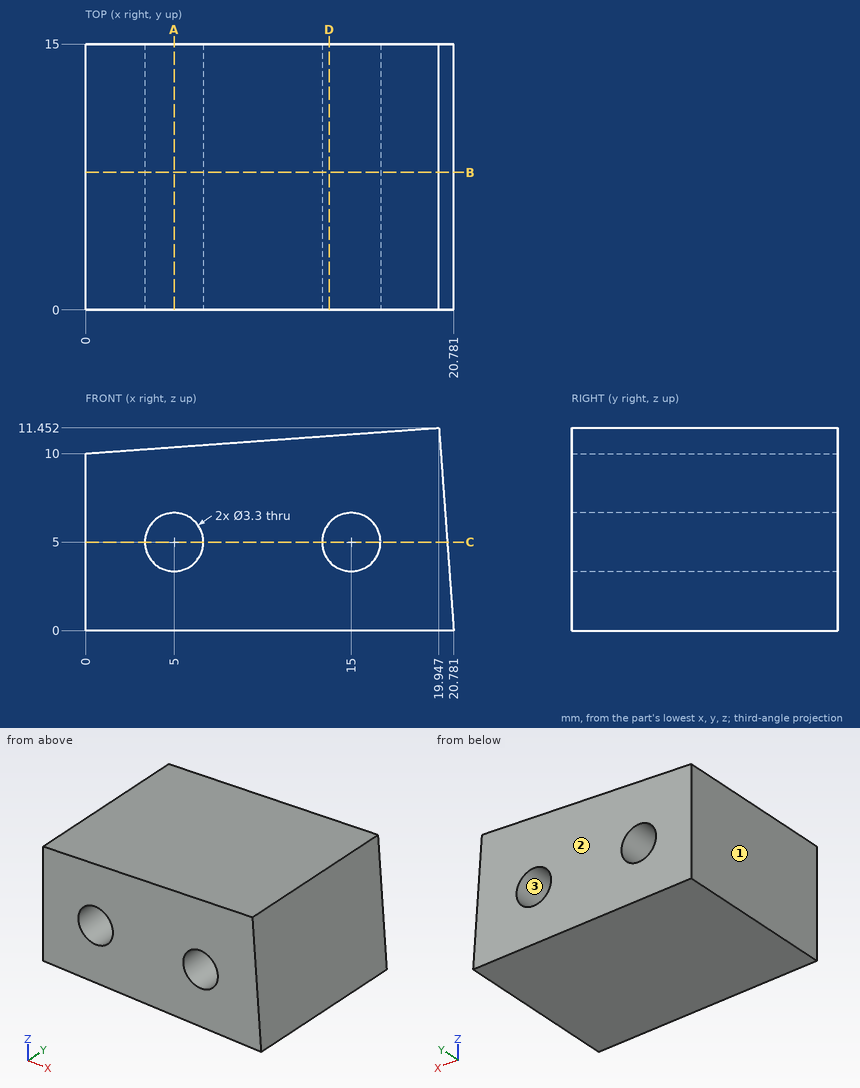
Design review of the part shown in the three views and the two pictorial views. Dimensions are in mm from the part's minimum x, y and z. Round coordinates to 2 decimals unless told otherwise and drop trailing zeros. Write each loop counter-clockwise with the first axis right and the second up, starting at its lowest first coordinate (ties: lowest second). Pieces come first, ordered by that corner, then holes. Notation, with made-up numbers: M 75,47.25 L 95,47.25 A16 cw 95,53.25 Z; hole C -22.75,62.25 d3. An arc over 180 degrees is marked long. One line per item, written item: value. Start each with the question number.
1. Take a section at A-A on x = 5. State the section outline as (y, z) points, then the cut area to 3 significant figures.
2. Take a section at C-C on z = 5. State the section outline as (x, y) points, then the cut area to 3 significant figures.
3. Draft analysis for pull direction X (two halves, no side actions). For the marked faces 1, 2 and 3, state which applies: pulls with the +X half, pulls with the -X half, needs draft (parallel to the pull), parting line crosses it, or undercut.
4. To check wall thickness, follow probe 1 along X at (y, z) = (4, 5); probe 2 along X at (y, z) = (11.25, 6.5) (1 decimal); probe 3 along Z at (x, y) = (4, 0.75). State the ranges of each line that lie inside material, in increasing order. Write a range as from..to.
5. Clearance check with flat-ended pins moving along their axes: P1, Ø1, axis at x = 5, y = 1.5, coming from the +Z side; P2, Ø4, axis at x = 10, y = 12, coming from the +Z side; P3, Ø5, axis at x = 9, y = 7, coming from the +Z side; P4, Ø2.5, axis at x = 15, z = 5, coming from the +Y side. State where each tip first meets the part, or that it passes through.
6. Take a section at D-D on x = 13.75. State the section outline as (y, z) points.
7. Take a section at B-B on y = 7.75. State the section outline as (x, z) points, then the cut area to 3 significant figures.
Computed:
1. outline: M 0,0 L 15,0 L 15,3.35 L 0,3.35 Z; M 0,6.65 L 15,6.65 L 15,10.36 L 0,10.36 Z
1. area: 106 mm²
2. outline: M 0,0 L 3.35,0 L 3.35,15 L 0,15 Z; M 6.65,0 L 13.35,0 L 13.35,15 L 6.65,15 Z; M 16.65,0 L 20.42,0 L 20.42,15 L 16.65,15 Z
2. area: 207 mm²
3. face 1: pulls with the -X half
3. face 2: needs draft
3. face 3: undercut
4. probe 1: x = 0..3.35, 6.65..13.35, 16.65..20.42
4. probe 2: x = 0..4.3, 5.7..14.3, 15.7..20.3
4. probe 3: z = 0..3.69, 6.31..10.29
5. P1: stops at z = 10.4
5. P2: stops at z = 10.87
5. P3: stops at z = 10.84
5. P4: passes through
6. outline: M 0,0 L 15,0 L 15,3.92 L 0,3.92 Z; M 0,6.08 L 15,6.08 L 15,11 L 0,11 Z
7. outline: M 0,0 L 20.78,0 L 19.95,11.45 L 0,10 Z; hole C 5,5 d3.3; hole C 15,5 d3.3
7. area: 202 mm²
